Read the model definition and answer for the solid it produces. Units are mm, in the model's axes. A direction names the side the tool comes from. Round coordinates to 2 decimals unless told otherwise and drop trailing zeros. Write each loop counter-clockwise with the first axis right and the second up, starting at its lowest first coordinate (ties: lowest second). Pieces come first, ordered by that corner, then holes. Notation, with made-up numbers: (11.5, 25) - (52.5, 25) arc R29 ccw to (52.5, 54) - close; hole circle Ø6 at (64.25, 69.5). An arc over 180 degrees is marked (long way). Use one line per item in the form item = value. Start each with the question number.
1) The part is cut by section B-B, the plane x = 10. Give the vertices of the cut face in (y, z).
2) For a pull along X with two mould halves and no side action, classify faces 1 (the face through (10, 7, 0)), 2 (the face through (10, 3, 6)), 3 (the face through (20, 1, 4)), 4 (the face through (5.864, 7.989, 2.127)) as released by +X, released by -X, zero draft, split by the parting line, or undercut.
3) For faces 5 (the face through (17.76, 7.35, 1.72)), 6 (the face through (14.024, 7.989, 2.163)), 7 (the face through (19, 4, 4.5)), determine the directions among +Z, -Z, +X, -X, +Y, -Y from which every point of the face is accessible in a straight line to the end or side of a thin tool.
4) Consider line 1 along Z through (x, y) = (15, 1.05); line 2 along X through (y, z) = (4.25, 4.25); line 3 along Z through (x, y) = (11.5, 7.5). Determine where each line is inside the solid, lowest interval first. Write a range as from..to.
5) The part is cut by section D-D, the plane z = 3.5. Give the vertices of the cut face in (x, y), plus the area to 3 significant figures.
6) The part is cut by section C-C, the plane y = 11.5. Give the vertices of the cut face in (x, z).
7) Each of these flat-tipped pins is pushed along its axis until it touches: pin 1 (2 mm diameter, centred on y = 11, z = 2.5, fed in from +X); pin 2 (3 mm diameter, centred on x = 15.5, z = 2.5, fed in from +Y); pin 3 (0.6 mm diameter, centred on x = 18.5, y = 5, fed in from +Z). Where does it stop, or does it pass through?
8) The part is cut by section A-A, the plane z = 5. Give the vertices of the cut face in (x, y).
Autodesk Inventor part; units mm, degrees
ref_plane "YZ Plane" through (0, 0, 0) normal (1, 0, 0) x (0, 1, 0)
ref_plane "XZ Plane" through (0, 0, 0) normal (0, 1, 0) x (-1, 0, 0)
ref_plane "XY Plane" through (0, 0, 0) normal (0, 0, 1) x (1, 0, 0)
sketch "Sketch1" plane through (0, 0, 0) normal (0, 0, 1) x (1, 0, 0)
  circle A0 centre (10, 11.5) radius 1.6
  line L0 (0, 0) -> (20.0001, 0)
  line L1 (0, 0) -> (0, 3)
  line L2 (20.0001, 0) -> (20.0001, 3)
  line L3 (0, 3) -> (16, 3) construction
  line L4 (20.0001, 3) -> (36.0001, 3) construction
  arc A1 (14.3301, 14) -> (5.6699, 14) centre (10, 11.5) ccw
  line L5 (10, 11.5) -> (5.6699, 14) construction
  line L6 (10, 11.5) -> (14.3301, 14) construction
  line L7 (5.6699, 14) -> (0, 3)
  line L8 (14.3301, 14) -> (20.0001, 3)
  dimension "d17" = 3
  dimension "d18" = 3
  dimension "d19" = 11.5
  dimension "d23" = 90
  dimension "d24" = 90
  dimension "d25" = 10
  dimension "d31" = 5
  dimension "d32" = 120
  dimension "d33" = 14
sketch "Sketch3" plane through (0, 0, 0) normal (0, 0, 1) x (1, 0, 0)
  point P0 (0, 0)
extrude "Extrusion1" add sketch "Sketch1" along normal blind 4.5
sketch "Sketch4" plane through (0, 0, 4.5) normal (0, 0, 1) x (1, 0, 0)
  line L0 (0, 3) -> (0, 0)
  line L1 (20.0001, 0) -> (20.0001, 3)
  line L2 (0, 0) -> (20.0001, 0)
  line L3 (20.0001, 0) -> (20.0001, 3)
  line L4 (3.884, 22.9404) -> (-0.9789, 3.2417)
  line L5 (20.0001, 3) -> (0, 3)
  line L6 (0, 3) -> (0, 0)
extrude "Extrusion2" add sketch "Sketch4" along normal blind 4.5
sketch "Sketch5" plane through (0, 0, 0) normal (0, -1, 0) x (1, 0, 0)
  circle A0 centre (5, 5) radius 0.5
  circle A1 centre (15, 5) radius 0.5
  line L0 (0, 0) -> (20.0001, 0)
  dimension "d13" = 1
  dimension "d14" = 1
  dimension "d38" = 5
  dimension "d39" = 5
extrude "Extrusion3" cut sketch "Sketch5" against normal blind 5.5
sketch "Sketch6" plane through (0, 3, 9) normal (0, 1, 0) x (1, 0, 0)
  circle A0 centre (5, 4) radius 0.5
  circle A1 centre (5, 4) radius 3
  circle A2 centre (15, 4) radius 0.5
  circle A3 centre (15, 4) radius 3
  line L0 (0, 9) -> (20.0001, 9)
  dimension "d34" = 6
  dimension "d35" = 6
  dimension "d40" = 5
  dimension "d41" = 5
extrude "Extrusion4" cut sketch "Sketch6" along normal up to next
properties part number "lower_deck_shaft_mount_for_AD"
Geometry results:
q1.outline = (0, 0) - (9.9, 0) - (9.9, 4.5) - (3, 4.5) - (3, 9) - (0, 9) - close; (13.1, 0) - (16.5, 0) - (16.5, 4.5) - (13.1, 4.5) - close
q2.face_1 = zero draft
q2.face_2 = undercut
q2.face_3 = released by +X
q2.face_4 = undercut
q3.face_5 = +Z, -Z, +X, +Y
q3.face_6 = +Z, +Y
q3.face_7 = +Z, +X, -X, +Y
q4.line_1 = 0..4.5, 5.5..9
q4.line_2 = 0.64..2.1, 7.9..12.1, 17.9..19.36
q4.line_3 = 0..4.5
q5.outline = (0, 0) - (20, 0) - (20, 3) - (17.6, 7.66) - (17.6, 3) - (12.4, 3) - (12.4, 15.89) arc R5 ccw to (7.6, 15.89) - (7.6, 3) - (2.4, 3) - (2.4, 7.66) - (0, 3) - close; hole circle Ø3.2 at (10, 11.5)
q5.area = 127 mm2
q6.outline = (4.38, 0) - (8.4, 0) - (8.4, 4.5) - (7.96, 4.5) arc R3 cw to (4.38, 2.06) - close; (11.6, 0) - (15.62, 0) - (15.62, 2.06) arc R3 cw to (12.04, 4.5) - (11.6, 4.5) - close
q7.pin_1 = 16.39
q7.pin_2 = 14.45
q7.pin_3 = 4.5
q8.outline = (0, 0) - (4.5, 0) - (4.5, 3) - (0, 3) - close; (5.5, 0) - (14.5, 0) - (14.5, 3) - (5.5, 3) - close; (15.5, 0) - (20, 0) - (20, 3) - (15.5, 3) - close
